Drawing for the job (mm, zero at the part's lowest x, y, z). A direction names the side the tool comes from. Give positions to 0.01 mm unless a question says otherwise; leave off trailing zeros. Loops run counter-clockwise (first coordinate to the right, second up) from the corner with the lowest first, then second, coordinate; pieces in that order, holes last.
1) Flat gauge pins, fed straight in: P1, Ø2.5, axis at y = 7.5, z = 17, coming from the +X side (3 decimals); P2, Ø16, axis at x = 7, z = 20.5, coming from the -Y side; P3, Ø17, axis at x = 49.5, z = 25.5, coming from the +Y side (3 decimals). Where does each tip first touch, or does it go through?
2) 3-axis set-ups, long thin cutter, end or side, ignore diameter. For the marked faces 1, 2 and 3: which of +Z, -Z, +X, -X, +Y, -Y reach the whole face in a straight line?
3) Band-saw the part on B-B on y = 15.25. List the corners of the cut face in (x, z), then the cut area to 3 significant figures.
4) Wall check: line 1 (X direction, y = 15.95, z = 10); line 2 (X direction, y = 14.9, z = 26); line 3 (X direction, y = 10.5, z = 25.5) (3 decimals). Give the ranges that are in metal, low to high.
5) Band-saw the part on A-A on z = 10. List the corners of the cut face in (x, y) (3 decimals).
6) Band-saw the part on D-D on y = 8.75. List the corners of the cut face in (x, z) (3 decimals).
7) Band-saw the part on C-C on x = 2.5. List the corners of the cut face in (y, z) (3 decimals).
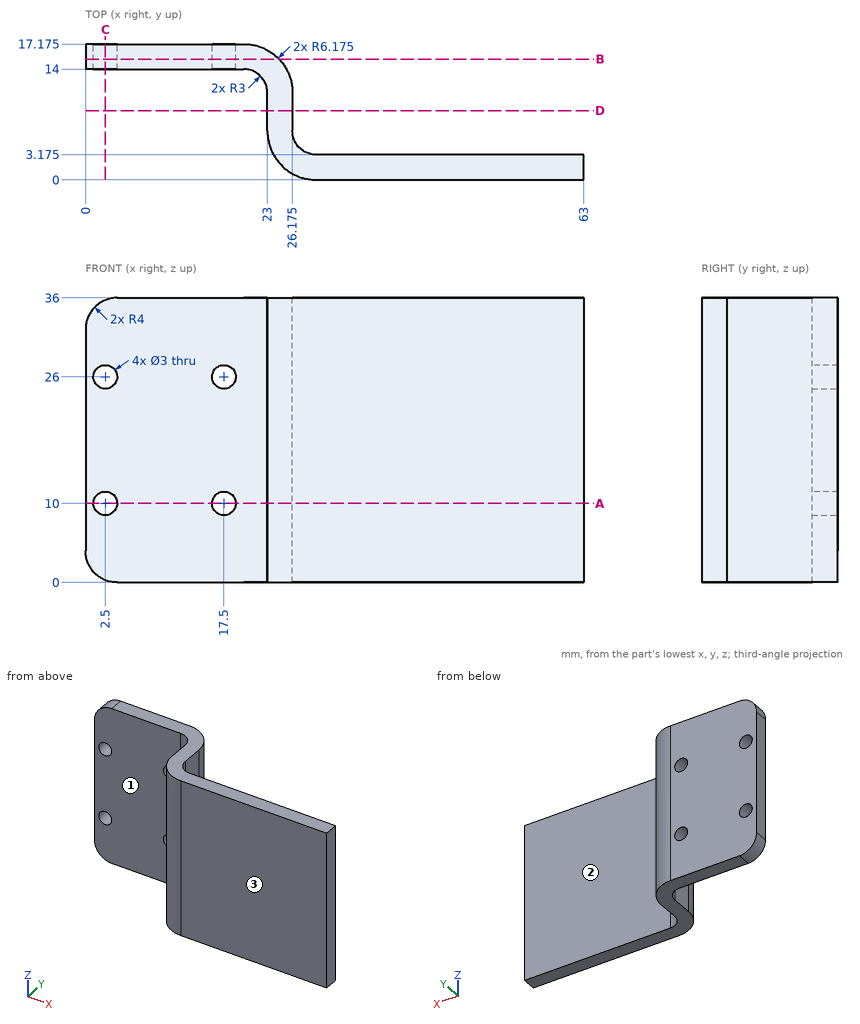
Findings below:
1. P1: stops at x = 26.175
1. P2: stops at y = 14
1. P3: stops at y = 3.175
2. face 1: +Z, -Z, -X, -Y
2. face 2: +Z, -Z, +X, +Y
2. face 3: +Z, -Z, +X, -X, -Y
3. outline: (0, 4) arc R4 ccw to (4, 0) - (24.48, 0) - (24.48, 36) - (4, 36) arc R4 ccw to (0, 32) - close; hole circle Ø3 at (2.5, 10); hole circle Ø3 at (2.5, 26); hole circle Ø3 at (17.5, 10); hole circle Ø3 at (17.5, 26)
3. area: 846 mm2
4. line 1: x = 0 to 1, 4 to 16, 19 to 23.69
4. line 2: x = 0 to 1, 4 to 16, 19 to 24.79
4. line 3: x = 23 to 26.175
5. outline: (0, 14) - (1, 14) - (1, 17.175) - (0, 17.175) - close; (4, 14) - (16, 14) - (16, 17.175) - (4, 17.175) - close; (19, 14) - (20, 14) arc R3 cw to (23, 11) - (23, 6.175) arc R6.175 ccw to (29.175, 0) - (63, 0) - (63, 3.175) - (29.175, 3.175) arc R3 cw to (26.175, 6.175) - (26.175, 11) arc R6.175 ccw to (20, 17.175) - (19, 17.175) - close
6. outline: (23, 0) - (26.175, 0) - (26.175, 36) - (23, 36) - close
7. outline: (14, 0.292) - (17.175, 0.292) - (17.175, 8.5) - (14, 8.5) - close; (14, 11.5) - (17.175, 11.5) - (17.175, 24.5) - (14, 24.5) - close; (14, 27.5) - (17.175, 27.5) - (17.175, 35.708) - (14, 35.708) - close
